from build123d import *

# Parameters (mm, degrees)
ESTRUSIONE_ESTRUSIONE1_DEPTH = 17
SCHIZZO2_R                   = 2
TAGLIO_ESTRUSIONE1_DEPTH     = 6.8


with BuildPart() as part:
    # Schizzo1 → Estrusione-Estrusione1 (new body)
    with BuildSketch(Plane.XY):
        Polygon((3, 0), (-3, 0), (-6, 3), (-6, 4), (-3, 4), (-3, 5.8), (3, 5.8), (3, 4), (6, 4), (6, 3), align=None)
    extrude(amount=ESTRUSIONE_ESTRUSIONE1_DEPTH)

    # Schizzo2 → Taglio-Estrusione1 (cut, through all)
    with BuildSketch(Plane(origin=(0, 5.8, 0), x_dir=(1, 0, 0), z_dir=(0, 1, 0))):
        with Locations((0, -6)):
            Circle(SCHIZZO2_R)
    extrude(amount=-TAGLIO_ESTRUSIONE1_DEPTH, mode=Mode.SUBTRACT)

    # Schizzo4 → Rivoluzione2 (revolve)
    with BuildSketch(Plane(origin=(0, 0, 0), x_dir=(0, 0, -1), z_dir=(1, 0, 0))):
        with BuildLine():
            Line((-12, -1.5), (-12, 0))
            Line((-12, 0), (-13.5, 0))
            ThreePointArc((-13.5, 0), (-13.060660172, -1.060660172), (-12, -1.5))
        make_face()
    revolve(axis=Axis((0, 0, 12), (0, -1, 0)))


solid = part.part
The listing builds one solid part. Answer for the finished solid, in the listing's coordinates (mm). A direction names the side the tool comes from. Coordinates: 2 decimals unless noted, no trailing zeros. Order: outer loops, then holes, each group sorted by start corner. A loop starts at its lowest first (then second) coordinate and runs counter-clockwise, first axis right, second up. Notation, with made-up numbers: (12, 80.5) -> (47, 80.5) arc R18 ccw to (47, 91.5) -> close; hole circle Ø9 at (-6.5, 24.5). An arc over 180 degrees is marked (long way). Answer in a Markdown table with one row per item. Add a question column.
Item 1: Find section A-A (z = 6). Write down the section's boundary in (x, y).
Item 2: Find the intervals of material crossed by L1, parallel to Z at x = 0, y = 2.05; L2, parallel to X at y = 3.25, z = 6; L3, parallel to Y at x = -2.75, z = 12.25, in increasing order. Write a range as from..to.
Item 3: Determine the mould class of faces 4 (the face through (0, 3, 8)), 5 (the face through (0, 3, 17)), 6 (the face through (-5, 4, 8)) for opening direction Z: +Z half, -Z half, draft (parallel to the pull), parting line (faces both ways), or undercut.
Item 4: Find section D-D (z = 15). Write down the section's boundary in (x, y).
Item 5: Each of these flat-tipped pins is pushed along its axis until it touches: P1, Ø2, axis at y = 1.5, z = 11.5, coming from the +X side; P2, Ø2, axis at y = 5.5, z = 6, coming from the -X side; P3, Ø0.9, axis at x = -5, z = 4.5, coming from the +Y side. Where does it stop, or does it pass through?
Item 6: Find section B-B (y = 2.75). Write down the section's boundary in (x, z), then the cut area to 3 significant figures.
Item 7: Find section C-C (x = 0). Write down the section's boundary in (y, z), then the cut area to 3 significant figures.
Item 8: Which of the six approach directions +Z, -Z, +X, -X, +Y, -Y give full straight-line access (tool end or side, diameter ignored) to faces 1 (the face through (6, 3.5, 8.4)), 2 (the face through (3, 5, 8)), 3 (the face through (-3, 5, 8))?
Result set:
| question | item | result |
|---|---|---|
| 1 | outline | (-6, 3) -> (-3, 0) -> (-2, 0) -> (-2, 5.8) -> (-3, 5.8) -> (-3, 4) -> (-6, 4) -> close; (2, 0) -> (3, 0) -> (6, 3) -> (6, 4) -> (3, 4) -> (3, 5.8) -> (2, 5.8) -> close |
| 2 | L1 | z = 0..4, 8..17 |
| 2 | L2 | x = -6..-2, 2..6 |
| 2 | L3 | y = 0..5.8 |
| 3 | face 4 | undercut |
| 3 | face 5 | +Z half |
| 3 | face 6 | draft |
| 4 | outline | (-6, 3) -> (-3, 0) -> (3, 0) -> (6, 3) -> (6, 4) -> (3, 4) -> (3, 5.8) -> (-3, 5.8) -> (-3, 4) -> (-6, 4) -> close |
| 5 | P1 | stops at x = 5.5 |
| 5 | P2 | stops at x = -3 |
| 5 | P3 | stops at y = 4 |
| 6 | outline | (-5.75, 0) -> (5.75, 0) -> (5.75, 17) -> (-5.75, 17) -> close; hole circle Ø4 at (0, 6) |
| 6 | area | 183 mm² |
| 7 | outline | (0, 0) -> (5.8, 0) -> (5.8, 4) -> (0, 4) -> close; (0, 8) -> (5.8, 8) -> (5.8, 17) -> (0, 17) -> (0, 13.5) arc R1.5 ccw to (0, 10.5) -> close |
| 7 | area | 78.9 mm² |
| 8 | face 1 | +Z, -Z, +X, +Y, -Y |
| 8 | face 2 | +Z, -Z, +X, +Y |
| 8 | face 3 | +Z, -Z, -X, +Y |
